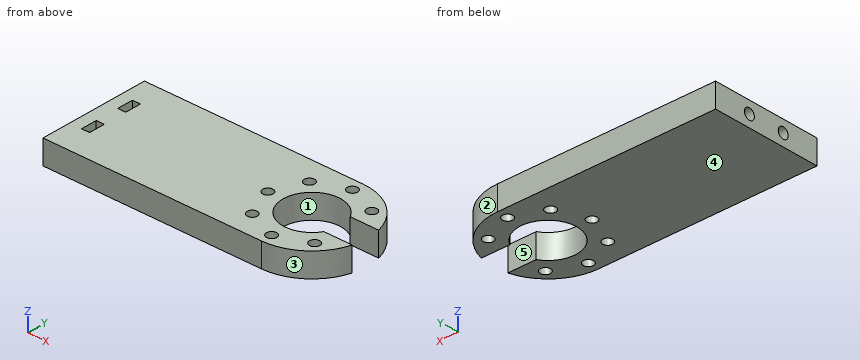
Autodesk Inventor part; units mm, degrees
ref_plane "YZ Plane" through (0, 0, 0) normal (1, 0, 0) x (0, 1, 0)
ref_plane "XZ Plane" through (0, 0, 0) normal (0, 1, 0) x (-1, 0, 0)
ref_plane "XY Plane" through (0, 0, 0) normal (0, 0, 1) x (1, 0, 0)
sketch "스케치1" plane through (0, 0, 0) normal (0, 0, 1) x (1, 0, 0)
  circle A0 centre (0, 0) radius 13.8
  circle A1 centre (0, 0) radius 7.2
  circle A2 centre (0, -11) radius 1.2813
  circle A3 centre (-7.7782, -7.7782) radius 1.2813
  circle A4 centre (-11, 0) radius 1.2813
  circle A5 centre (-7.7782, 7.7782) radius 1.2813
  circle A6 centre (0, 11) radius 1.2813
  circle A7 centre (7.7782, 7.7782) radius 1.2813
  circle A8 centre (11, 0) radius 1.2813
  circle A9 centre (7.7782, -7.7782) radius 1.2813
  circle A10 centre (0, 0) radius 3.15
  circle A11 centre (0, 0) radius 3.5972
  line L0 (0, -3.5972) -> (0, 3.5972)
  line L1 (0, 3.5972) -> (17.7956, 3.5972)
  line L2 (17.7956, 3.5972) -> (17.7956, -3.5972)
  line L3 (17.7956, -3.5972) -> (0, -3.5972)
  line L4 (-54.4347, 13.8) -> (-54.4347, -13.8)
  line L5 (0, -13.8) -> (0, 13.8)
  line L6 (0, 13.8) -> (-54.4347, 13.8)
  line L7 (-54.4347, 13.8) -> (-54.4347, -13.8)
  line L8 (-54.4347, -13.8) -> (0, -13.8)
  point P0 (0, 0)
  point P1 (6.237, 3.5972)
  point P2 (13.3229, 3.5972)
  point P3 (13.3229, -3.5972)
  point P4 (6.237, -3.5972)
extrude "돌출1" add sketch "스케치1" along normal blind 6 contours L5 A6 A1 A2 A0 | A0 L1 A1 L5 A6 | A0 L8 L4 L6 | L5 A2 A1 L3 A0
sketch "스케치2" plane through (-54.4347, -13.8, 0) normal (-1, 0, 0) x (0, 0, 1)
  line L0 (0, 13.8) -> (6, 13.8)
  line L1 (6, 15.0812) -> (6, 12.5187)
  line L2 (0, 13.8) -> (3, 13.8)
  line L3 (3, 13.8) -> (3, 0)
  line L4 (0, 0) -> (6, 0)
  line L5 (3, 0) -> (3, 9.2)
  line L6 (3, 9.2) -> (3, 18.4)
  circle A0 centre (3, 18.4) radius 1.35
  circle A1 centre (3, 9.2) radius 1.35
  dimension "d2" = 3
  dimension "d3" = 9.2
  dimension "d4" = 9.2
  dimension "d5" = 2.7
  dimension "d6" = 2.7
extrude "돌출2" cut sketch "스케치2" against normal blind 3
sketch "스케치3" plane through (0, 0, 6) normal (0, 0, 1) x (1, 0, 0)
  line L0 (-50.4347, -2.45) -> (-50.4347, -6.45)
  line L1 (-50.4347, 7.3745) -> (-50.4347, 3.3745)
  line L2 (-54.4347, 13.8) -> (-54.4347, -13.8)
  line L3 (-54.4347, 5.2526) -> (-50.4347, 5.2526)
  line L4 (-54.4347, -4.5845) -> (-50.4347, -4.5845)
  line L5 (-51.4347, -2.5845) -> (-51.4347, -6.5845)
  line L6 (-51.4347, -6.5845) -> (-49.4347, -6.5845)
  line L7 (-49.4347, -6.5845) -> (-49.4347, -2.5845)
  line L8 (-49.4347, -2.5845) -> (-51.4347, -2.5845)
  line L9 (-51.4347, -2.5845) -> (-49.4347, -6.5845) construction
  line L10 (-51.4347, -6.5845) -> (-49.4347, -2.5845) construction
  line L11 (-51.4347, 7.2526) -> (-51.4347, 3.2526)
  line L12 (-51.4347, 3.2526) -> (-49.4347, 3.2526)
  line L13 (-49.4347, 3.2526) -> (-49.4347, 7.2526)
  line L14 (-49.4347, 7.2526) -> (-51.4347, 7.2526)
  line L15 (-51.4347, 7.2526) -> (-49.4347, 3.2526) construction
  line L16 (-51.4347, 3.2526) -> (-49.4347, 7.2526) construction
  point P0 (0, 0)
  dimension "d9" = 4
  dimension "d10" = 2
  dimension "d11" = 4
  dimension "d12" = 2
extrude "돌출3" cut sketch "스케치3" against normal blind 4
properties part number "_thigh_adt_body"
Can you work these out from the model? Positions are in its coordinate system, mm. Face numbers are marked on the shaded views. A direction names the side the tool comes from. Coordinates: 2 decimals unless noted, no trailing zeros. Loops run counter-clockwise (first coordinate to the right, second up) from the corner with the lowest first, then second, coordinate; pieces in that order, holes last. Notation, with made-up numbers: M 10,-27 L 21,-27 A21 ccw 21,-23 Z; hole C 83,-21.5 d7. An arc over 180 degrees is marked long. Put each result on its own line as item: value. Start each with the question number.
(1) Imagine slicing it at A-A on x = -11. List the corners of the cut face in (y, z) for me.
(2) I need wall thicknesses on probe 1 along Y at (x, z) = (0, 4.1); probe 2 along Y at (x, z) = (-52.3, 3); probe 3 along Y at (x, z) = (1, 4.75). Which ranges of each line are inside material? Lowest first, please.
(3) We'd pull the mould along Y, two halves only. Please class the marked faces 1, 2 and 3: +Y half, -Y half, draft (parallel to the pull), parting line (faces both ways), or undercut.
(4) Imagine slicing it at B-B on y = 0. List the corners of the cut face in (x, z) for me.
(5) Will these pins go through, and if not, where does the flat tip stop? pin 1 Ø3 at (y, z) = (9.5, 1) entering from +X; pin 2 Ø2.5 at (x, y) = (0, 11) entering from -Z.
(6) Imagine slicing it at D-D on z = 0.6. List the corners of the cut face in (x, y) for me, and give its area (3 significant figures).
(7) Which directions (+Z, -Z, +X, -X, +Y, -Y) give clear straight access to the entire face, cutting with the end or side of a thin tool? Please do the marked faces 4 and 5.
(8) Imagine slicing it at C-C on y = -4.6. List the corners of the cut face in (x, z) for me.
Worked answers:
1. outline: M -13.8,0 L -1.28,0 L -1.28,6 L -13.8,6 Z; M 1.28,0 L 13.8,0 L 13.8,6 L 1.28,6 Z
2. probe 1: y = -13.8 to -12.28, -9.72 to -7.2, 7.2 to 9.72, 12.28 to 13.8
2. probe 2: y = -13.8 to -5.95, -3.25 to 3.25, 5.95 to 13.8
2. probe 3: y = -13.76 to -11.8, -10.2 to -7.13, 7.13 to 10.2, 11.8 to 13.76
3. face 1: undercut
3. face 2: +Y half
3. face 3: -Y half
4. outline: M -54.43,0 L -12.28,0 L -12.28,6 L -54.43,6 Z; M -9.72,0 L -7.2,0 L -7.2,6 L -9.72,6 Z
5. pin 1: stops at x = 11.24
5. pin 2: passes through
6. outline: M -54.43,-13.8 L 0,-13.8 A13.8 ccw 13.32,-3.6 L 6.24,-3.6 A7.2 cw long 6.24,3.6 L 13.32,3.6 A13.8 ccw 0,13.8 L -54.43,13.8 Z; hole C -11,0 d2.56; hole C -7.78,-7.78 d2.56; hole C -7.78,7.78 d2.56; hole C 0,-11 d2.56; hole C 0,11 d2.56; hole C 7.78,-7.78 d2.56; hole C 7.78,7.78 d2.56
6. area: 1,550 mm2
7. face 4: -Z, +X, -X, +Y, -Y
7. face 5: +Z, -Z, +X
8. outline: M -54.43,0 L -5.54,0 L -5.54,6 L -49.43,6 L -49.43,2 L -51.43,2 L -51.43,1.65 L -54.43,1.65 Z; M -54.43,4.35 L -51.43,4.35 L -51.43,6 L -54.43,6 Z; M 5.54,0 L 13.01,0 L 13.01,6 L 5.54,6 Z
